Here's the drawing with two shaded views (mm, measured from the low corner). I have some questions. A direction names the side the tool comes from. Coordinates: 2 decimals unless noted, no trailing zeros. Loops run counter-clockwise (first coordinate to the right, second up) from the corner with the lowest first, then second, coordinate; pieces in that order, holes last. Notation, with made-up numbers: (29, 32) - (86, 32) arc R19 ccw to (86, 53) - close; hole circle Ø6 at (68.5, 46.5). An arc over 180 degrees is marked (long way). One line per item, written item: value. Start each with the question number.
(1) If we section it at A-A on z = 9: Write out the boundary of the cut face in (x, y).
(2) If I drill on line 1 along Z through (x, y) = (9, 4.55); line 2 along Y through (x, z) = (5.5, 2.25), over which ranges is the centre line in solid material (lowest first)? Write a range as from..to.
(3) If we mould it in two halves opening along X, with no side actions, what happens to the marked faces 3, 4 and 5? For each: pulls with the +X half, pulls with the -X half, needs draft (parallel to the pull), parting line crosses it, or undercut.
(4) If we section it at C-C on x = 9: Write out the boundary of the cut face in (y, z), then the cut area to 3 significant figures.
(5) If we section it at D-D on y = 0.85: Write out the boundary of the cut face in (x, z).
(6) I'm going to push flat-ended pins straight in: P1, Ø9, axis at x = 9, z = 9, coming from the +Y side; P2, Ø1, axis at x = 13.5, y = 4, coming from the +Z side; P3, Ø3.5, axis at x = 9, z = 9, coming from the +Y side; P4, Ø1.5, axis at y = 1.5, z = 6.5, coming from the +X side. Where does each tip first touch, or does it pass through?
(7) On a 3-axis mill with a long thin cutter (end or side, diameter ignored), from which of +Z, -Z, +X, -X, +Y, -Y can I reach the whole of each face in a straight line? I mean the marked faces 1 and 2. Say none if no direction works.
(8) If we section it at B-B on y = 4.35: Write out the boundary of the cut face in (x, z).
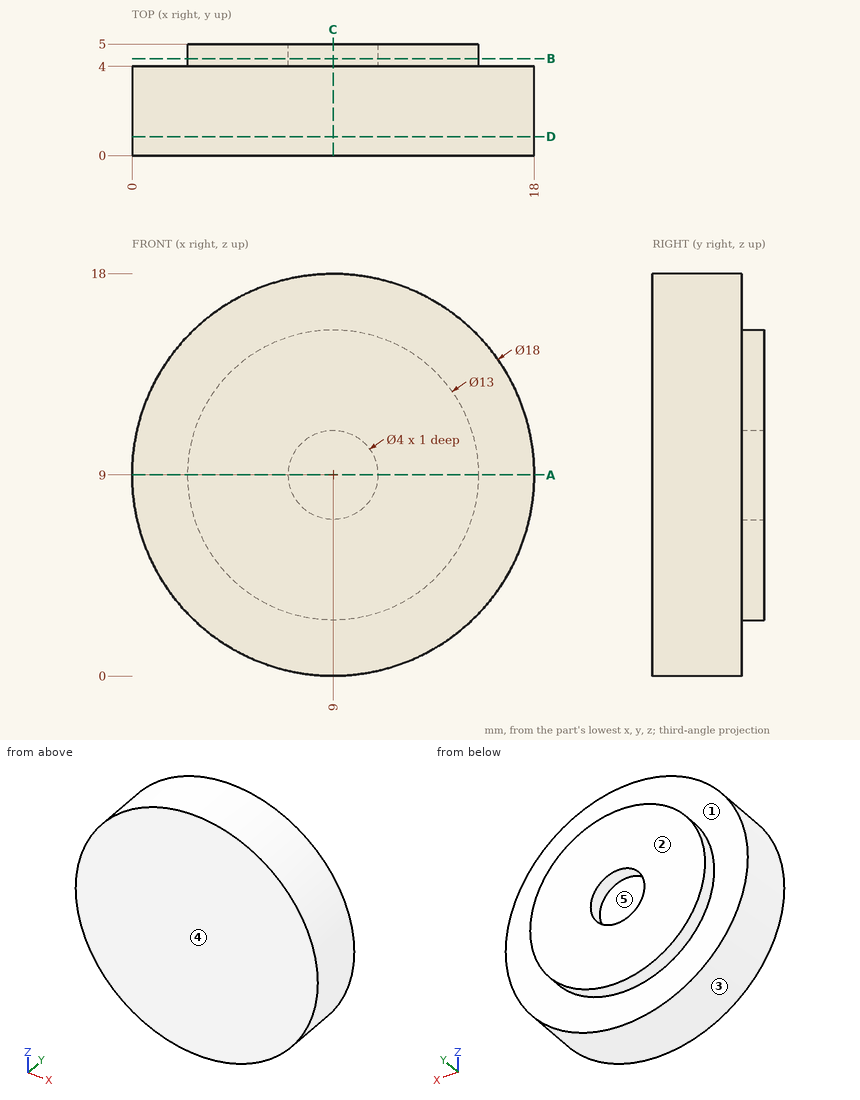
Values:
1. outline: (0, 0) - (18, 0) - (18, 4) - (15.5, 4) - (15.5, 5) - (11, 5) - (11, 4) - (7, 4) - (7, 5) - (2.5, 5) - (2.5, 4) - (0, 4) - close
2. line 1: z = 2.5..7, 11..15.5
2. line 2: y = 0..4
3. face 3: parting line crosses it
3. face 4: needs draft
3. face 5: undercut
4. outline: (0, 0) - (4, 0) - (4, 2.5) - (5, 2.5) - (5, 7) - (4, 7) - (4, 11) - (5, 11) - (5, 15.5) - (4, 15.5) - (4, 18) - (0, 18) - close
4. area: 81.0 mm2
5. outline: circle Ø18 at (9, 9)
6. P1: stops at y = 5
6. P2: stops at z = 17.06
6. P3: stops at y = 4
6. P4: stops at x = 17.83
7. face 1: +Y
7. face 2: +Z, -Z, +X, -X, +Y
8. outline: circle Ø13 at (9, 9); hole circle Ø4 at (9, 9)
